Print and shaded views of the part. All mm, measured from the part's lowest x, y and z. A direction names the side the tool comes from. Round coordinates to 2 decimals unless told otherwise and drop trailing zeros. Order: outer loops, then holes, each group sorted by start corner. A loop starts at its lowest first (then second) coordinate and runs counter-clockwise, first axis right, second up. Notation, with made-up numbers: (80.25, -4.75) -> (131.25, -4.75) arc R17 ccw to (131.25, 8.25) -> close; hole circle Ø2 at (53, 32.25). An arc over 180 degrees is marked (long way). Answer as CSV lines item,"result".
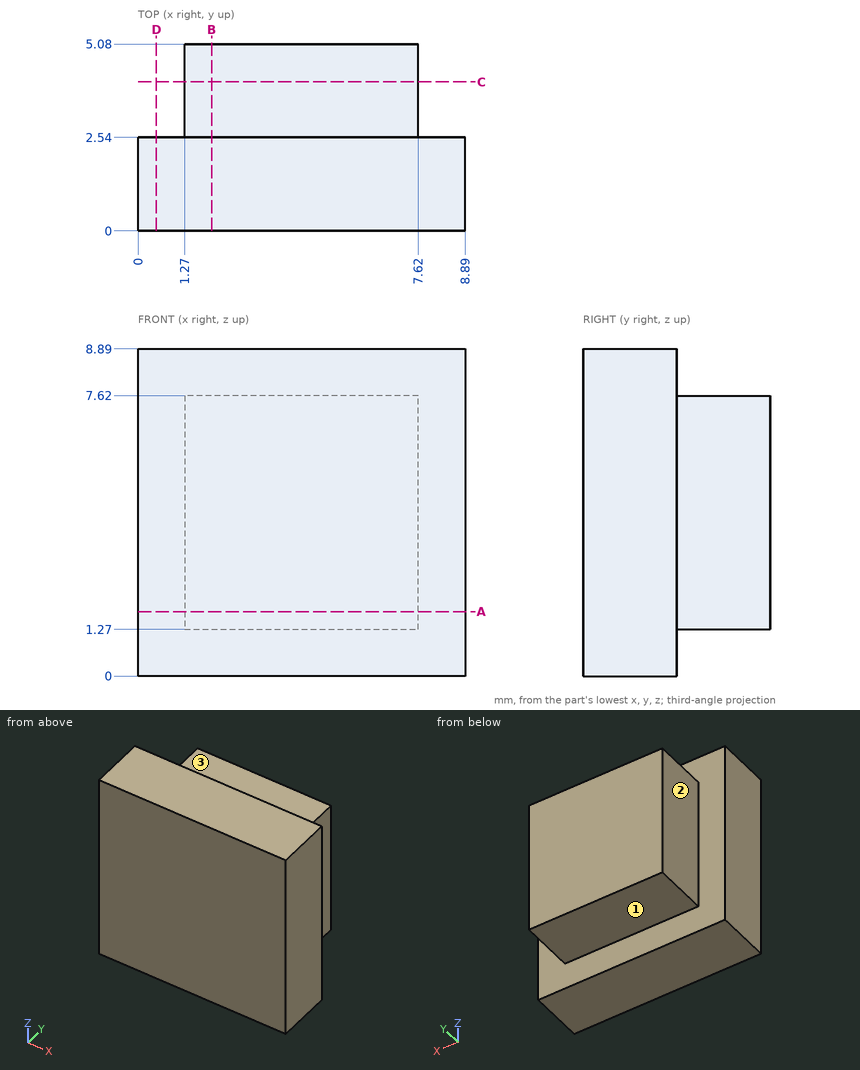
Q1. Saw through at A-A (z = 1.75). Write the cut outline in (x, y).
Checks:
outline,"(0, 0) -> (8.89, 0) -> (8.89, 2.54) -> (7.62, 2.54) -> (7.62, 5.08) -> (1.27, 5.08) -> (1.27, 2.54) -> (0, 2.54) -> close"
Q2. Wall check: L1, parallel to Y at x = 0.5, z = 2.5; L2, parallel to X at y = 3.2, z = 5. Give the ranges that are in metal, low to high. Write a range as [from, to].
Checks:
L1,"[0, 2.54]"
L2,"[1.27, 7.62]"
Q3. Saw through at B-B (x = 2). Write the cut outline in (y, z).
Checks:
outline,"(0, 0) -> (2.54, 0) -> (2.54, 1.27) -> (5.08, 1.27) -> (5.08, 7.62) -> (2.54, 7.62) -> (2.54, 8.89) -> (0, 8.89) -> close"
Q4. Tool access for the marked faces 1, 2 and 3: list every direction of +Z, -Z, +X, -X, +Y, -Y with a clear straight run to the whole face (end or side of a thin tool).
Checks:
face 1,"-Z, +X, -X, +Y"
face 2,"+Z, -Z, -X, +Y"
face 3,"+Z, +X, -X, +Y"
Q5. Saw through at D-D (x = 0.5). Write the cut outline in (y, z), plus the area to 3 significant figures.
Checks:
outline,"(0, 0) -> (2.54, 0) -> (2.54, 8.89) -> (0, 8.89) -> close"
area,"22.6 mm²"
Q6. Saw through at C-C (y = 4.05). Write the cut outline in (x, z), plus the area to 3 significant figures.
Checks:
outline,"(1.27, 1.27) -> (7.62, 1.27) -> (7.62, 7.62) -> (1.27, 7.62) -> close"
area,"40.3 mm²"
Q7. Flat gauge pin, fed straight in: pin 1 (2 mm diameter, centred on x = 5, y = 4.5, fed in from +Z). Where does the tip first touch, or does it go through?
Checks:
pin 1,"z = 7.62"
